Work out the finished part from the listing and answer in its coordinate system (mm). A direction names the side the tool comes from. Round coordinates to 2 decimals unless told otherwise and drop trailing zeros. Write each loop counter-clockwise with the first axis right and the second up, starting at its lowest first coordinate (ties: lowest second). Pieces come first, ordered by that corner, then holes. Notation, with made-up numbers: (-36.75, 84) - (2.25, 84) arc R18 ccw to (2.25, 93) - close; hole circle Ø2 at (33, 44.5). An arc over 180 degrees is marked (long way). Answer as a JSON object with one key per item and string values.
```python
from build123d import *

# Parameters (mm, degrees)
SKETCH1_W           = 68
SKETCH1_H           = 68
SKETCH1_W_2         = 2
SKETCH1_H_2         = 5
SKETCH1_R           = 5
BOSS_EXTRUDE1_DEPTH = 2
FILLET2_R           = 5
FILLET3_R           = 5
FILLET4_R           = 5
FILLET5_R           = 5
SKETCH2_W           = 3
SKETCH2_H           = 5
CUT_EXTRUDE1_DEPTH  = 10


with BuildPart() as part:
    # Sketch1 → Boss-Extrude1 (new body)
    with BuildSketch(Plane.XY):
        Rectangle(SKETCH1_W, SKETCH1_H)
        with Locations((-29, -27.5)):
            Rectangle(SKETCH1_W_2, SKETCH1_H_2, mode=Mode.SUBTRACT)
        with Locations((0, -25)):
            Circle(SKETCH1_R, mode=Mode.SUBTRACT)
        with Locations((29, -27.5)):
            Rectangle(SKETCH1_W_2, SKETCH1_H_2, mode=Mode.SUBTRACT)
        with Locations((-28, 0)):
            Circle(SKETCH1_R, mode=Mode.SUBTRACT)
        with Locations((-29, 27.5)):
            Rectangle(SKETCH1_W_2, SKETCH1_H_2, mode=Mode.SUBTRACT)
        with BuildLine():
            ThreePointArc((-12, -2.5), (-14.5, 0), (-12, 2.5))
            Line((-12, 2.5), (-2.5, 2.5))
            Line((-2.5, 2.5), (-2.5, 12))
            ThreePointArc((-2.5, 12), (0, 14.5), (2.5, 12))
            Line((2.5, 12), (2.5, 2.5))
            Line((2.5, 2.5), (12, 2.5))
            ThreePointArc((12, 2.5), (14.5, 0), (12, -2.5))
            Line((12, -2.5), (2.5, -2.5))
            Line((2.5, -2.5), (2.5, -12))
            ThreePointArc((2.5, -12), (0, -14.5), (-2.5, -12))
            Line((-2.5, -12), (-2.5, -2.5))
            Line((-2.5, -2.5), (-12, -2.5))
        make_face(mode=Mode.SUBTRACT)
        with Locations((28, 0)):
            Circle(SKETCH1_R, mode=Mode.SUBTRACT)
        with Locations((0, 25)):
            Circle(SKETCH1_R, mode=Mode.SUBTRACT)
        with Locations((29, 27.5)):
            Rectangle(SKETCH1_W_2, SKETCH1_H_2, mode=Mode.SUBTRACT)
    extrude(amount=BOSS_EXTRUDE1_DEPTH)

    # Fillet2
    fillet2_edges = [part.edges().sort_by_distance(p)[0] for p in [
        (34, 34, 1),
    ]]
    fillet(fillet2_edges, radius=FILLET2_R)

    # Fillet3
    fillet3_edges = [part.edges().sort_by_distance(p)[0] for p in [
        (-34, 34, 1),
    ]]
    fillet(fillet3_edges, radius=FILLET3_R)

    # Fillet4
    fillet4_edges = [part.edges().sort_by_distance(p)[0] for p in [
        (-34, -34, 1),
    ]]
    fillet(fillet4_edges, radius=FILLET4_R)

    # Fillet5
    fillet5_edges = [part.edges().sort_by_distance(p)[0] for p in [
        (34, -34, 1),
    ]]
    fillet(fillet5_edges, radius=FILLET5_R)

    # Sketch2 → Cut-Extrude1 (cut)
    with BuildSketch(Plane.XY.offset(2)):
        with Locations((29, 27.5)):
            Rectangle(SKETCH2_W, SKETCH2_H)
        with Locations((-29, 27.5)):
            Rectangle(SKETCH2_W, SKETCH2_H)
        with Locations((29, -27.5)):
            Rectangle(SKETCH2_W, SKETCH2_H)
        with Locations((-29, -27.5)):
            Rectangle(SKETCH2_W, SKETCH2_H)
    extrude(amount=-CUT_EXTRUDE1_DEPTH, mode=Mode.SUBTRACT)


solid = part.part
```
Item 1: A cutting plane is placed at D-D (z = 1.15). Give the number of separate pieces and of enclosed holes in the cut face, and give its area (3 significant figures).
Results found:
{"separate pieces": "1", "enclosed holes": "9", "area": "3,970 mm²"}
Item 2: A cutting plane is placed at C-C (y = 0). Write down the section's boundary in (x, z), and give its area (3 significant figures).
Results found:
{"outline": "(-34, 0) - (-33, 0) - (-33, 2) - (-34, 2) - close; (-23, 0) - (-14.5, 0) - (-14.5, 2) - (-23, 2) - close; (14.5, 0) - (23, 0) - (23, 2) - (14.5, 2) - close; (33, 0) - (34, 0) - (34, 2) - (33, 2) - close", "area": "38.0 mm²"}
Item 3: A cutting plane is placed at A-A (y = -28). Write down the section's boundary in (x, z).
Results found:
{"outline": "(-34, 0) - (-30.5, 0) - (-30.5, 2) - (-34, 2) - close; (-27.5, 0) - (-4, 0) - (-4, 2) - (-27.5, 2) - close; (4, 0) - (27.5, 0) - (27.5, 2) - (4, 2) - close; (30.5, 0) - (34, 0) - (34, 2) - (30.5, 2) - close"}
Item 4: A cutting plane is placed at B-B (x = -26.5). Write down the section's boundary in (y, z), and give its area (3 significant figures).
Results found:
{"outline": "(-34, 0) - (-4.77, 0) - (-4.77, 2) - (-34, 2) - close; (4.77, 0) - (34, 0) - (34, 2) - (4.77, 2) - close", "area": "117 mm²"}
Item 5: Consider line 1 along Y through (x, z) = (-28, 1.45); line 2 along Y through (x, z) = (0, 0.6); line 3 along X through (y, z) = (11, 0.1). Determine where each line is inside the solid, lowest interval first.
Results found:
{"line 1": "-34 to -30, -25 to -5, 5 to 25, 30 to 34", "line 2": "-34 to -30, -20 to -14.5, 14.5 to 20, 30 to 34", "line 3": "-34 to -2.5, 2.5 to 34"}
Item 6: This flat-tipped pin is pushed along its axis until it touches: P1, Ø0.6, axis at x = 29.5, z = 1, coming from the +Y side. Where does it stop, or does it pass through?
Results found:
{"P1": "y = 34"}
Item 7: Determine the mould class of faces 3 (the cylindrical face through (-32, 33, 1)), 4 (the flat face through (29, 25, 1)), 5 (the cylindrical face through (32, -33, 1)), 6 (the flat face through (-8, 8, 2)) for opening direction Y: pulls with the +Y half, pulls with the -Y half, needs draft (parallel to the pull), parting line crosses it, or undercut.
Results found:
{"face 3": "pulls with the +Y half", "face 4": "undercut", "face 5": "pulls with the -Y half", "face 6": "needs draft"}
Item 8: For faces 1 (the flat face through (-8, 8, 0)), 2 (the cylindrical face through (14.5, 0.1, 1)), determine the directions among +Z, -Z, +X, -X, +Y, -Y from which every point of the face is accessible in a straight line to the end or side of a thin tool.
Results found:
{"face 1": "-Z, +X, -X, +Y, -Y", "face 2": "+Z, -Z"}
